Part model, mm, in its own coordinate system. A direction names the side the tool comes from. Coordinates: 2 decimals unless noted, no trailing zeros. Loops run counter-clockwise (first coordinate to the right, second up) from the corner with the lowest first, then second, coordinate; pieces in that order, holes last. Notation, with made-up numbers: M 58,59 L 105,59 A25 cw 105,93 Z; hole C 37.25,22.25 d2. An arc over 180 degrees is marked long. Use a Markdown table: item, result. Add a question column.
1) Pin check, flat tips, straight feed: pin 1 Ø9.5 at (x, y) = (-57, -0.5) entering from +Z; pin 2 Ø6 at (x, y) = (-46.5, 99) entering from +Z; pin 3 Ø10 at (x, y) = (-109.5, 230) entering from -Z. Stop position of each tip, or through.
2) Band-saw the part on D-D (y = 132.5). List the corners of the cut face in (x, z).
3) Band-saw the part on B-B (x = -59.69). List the corners of the cut face in (y, z) (3 decimals), plus the area to 3 significant figures.
4) Tool access for faces 5 (the flat face through (342.9, 253, 42)), 6 (the cylindrical face through (50.605, -2.861, 18.21)), 7 (the flat face through (-293, 203.2, 54)), 8 (the cylindrical face through (-248.94, 254.71, 89.28)): list every direction of +Z, -Z, +X, -X, +Y, -Y with a clear straight run to the whole face (end or side of a thin tool).
5) Wall check: probe 1 along X at (y, z) = (184, -64); probe 2 along Y at (x, z) = (0, 12.5); probe 3 along X at (y, z) = (284.5, 32.5). Give the ranges that are in metal, low to high. Write a range as from..to.
6) Band-saw the part on A-A (z = -78.5). List the corners of the cut face in (x, y), plus the area to 3 significant figures.
7) Band-saw the part on C-C (y = 59.69). List the corners of the cut face in (x, z) (3 decimals), plus the area to 3 significant figures.
8) Pull direction X, two halves, no side cores. Call faces 1 (the cylindrical face through (-248.94, -62.79, 89.28)), 2 (the flat face through (-342.9, 253, 42)), 3 (the flat face through (-293, -12.7, 54)), 4 (the flat face through (-6, 98, 0)): released by +X, released by -X, zero draft, split by the parting line, or undercut.
from build123d import *

# Parameters (mm, degrees)
F0_W     = 914.4
F0_H     = 419.1
F1_DEPTH = 12.7
F2_R     = 36.83
F3_DEPTH = 12.7
F4_R     = 9.525
F5_DEPTH = 11.176
F6_W     = 101.6
F6_H     = 101.6
F7_DEPTH = 83.82
F8_W     = 12.7
F8_H     = 419.1
F9_DEPTH = 254
F10_R    = 25.4


with BuildPart() as f1:
    # F0 (on Top) → F1 (new body)
    with BuildSketch(Plane.XY):
        with Locations((0, 95.25)):
            Rectangle(F0_W, F0_H)
    extrude(amount=F1_DEPTH)

    # F2 (on face) → F3 (cut)
    with BuildSketch(Plane.XY.offset(12.7)):
        Circle(F2_R)
    extrude(amount=-F3_DEPTH, mode=Mode.SUBTRACT)

    # F4 (on face) → F5 (join)
    with BuildSketch(Plane.XY.offset(12.7)):
        with BuildLine():
            ThreePointArc((9.525, 59.69), (-6.7351920908, 66.4251920908), (0, 50.165))
            ThreePointArc((0, 50.165), (6.7351920908, 52.9548079092), (9.525, 59.69))
        make_face()
        with BuildLine():
            Line((36.83, 0), (48.26, 0))
            ThreePointArc((48.26, 0), (34.1249732601, 34.1249732601), (0, 48.26))
            Line((0, 48.26), (0, 36.83))
            ThreePointArc((0, 36.83), (26.0427427511, 26.0427427511), (36.83, 0))
        make_face()
        with BuildLine():
            Line((0, 36.83), (0, 48.26))
            ThreePointArc((0, 48.26), (-34.1249732601, 34.1249732601), (-48.26, 0))
            Line((-48.26, 0), (-36.83, 0))
            ThreePointArc((-36.83, 0), (-26.0427427511, 26.0427427511), (0, 36.83))
        make_face()
        with BuildLine():
            ThreePointArc((-48.26, 0), (-34.1249732601, -34.1249732601), (0, -48.26))
            Line((0, -48.26), (0, -36.83))
            ThreePointArc((0, -36.83), (-26.0427427511, -26.0427427511), (-36.83, 0))
            Line((-36.83, 0), (-48.26, 0))
        make_face()
        with BuildLine():
            ThreePointArc((0, -48.26), (34.1249732601, -34.1249732601), (48.26, 0))
            Line((48.26, 0), (36.83, 0))
            ThreePointArc((36.83, 0), (26.0427427511, -26.0427427511), (0, -36.83))
            Line((0, -36.83), (0, -48.26))
        make_face()
        with Locations((-59.69, 0)):
            Circle(F4_R)
        with BuildLine():
            ThreePointArc((9.525, -59.69), (6.7351920908, -52.9548079092), (0, -50.165))
            ThreePointArc((0, -50.165), (-6.7351920908, -66.4251920908), (9.525, -59.69))
        make_face()
        with BuildLine():
            ThreePointArc((69.215, 0), (59.69, 9.525), (50.165, 0))
            ThreePointArc((50.165, 0), (59.69, -9.525), (69.215, 0))
        make_face()
    extrude(amount=F5_DEPTH)

    # F6 (on face) → F7 (join)
    with BuildSketch(Plane.XY.offset(12.7)):
        with Locations((-292.1, 254)):
            Rectangle(F6_W, F6_H)
        with Locations((-292.1, -63.5)):
            Rectangle(F6_W, F6_H)
        with Locations((292.1, -63.5)):
            Rectangle(F6_W, F6_H)
        with Locations((292.1, 254)):
            Rectangle(F6_W, F6_H)
    extrude(amount=F7_DEPTH)

    # F8 (on face) → F9 (join)
    with BuildSketch(Plane(origin=(0, 0, 0), x_dir=(1, 0, 0), z_dir=(0, 0, -1))):
        with Locations((-450.85, -95.25)):
            Rectangle(F8_W, F8_H)
        with Locations((450.85, -95.25)):
            Rectangle(F8_W, F8_H)
    extrude(amount=F9_DEPTH)

    # F10
    f10_edges = [f1.edges().sort_by_distance(p)[0] for p in [
        (-342.9, -63.5, 96.52),
        (-342.9, 254, 96.52),
        (-241.3, 254, 96.52),
        (-241.3, -63.5, 96.52),
        (241.3, -63.5, 96.52),
        (241.3, 254, 96.52),
        (342.9, 254, 96.52),
        (342.9, -63.5, 96.52),
    ]]
    fillet(f10_edges, radius=F10_R)


solid = f1.part
Entries:
| question | item | result |
|---|---|---|
| 1 | pin 1 | z = 23.88 |
| 1 | pin 2 | z = 12.7 |
| 1 | pin 3 | z = 0 |
| 2 | outline | M -457.2,-254 L -444.5,-254 L -444.5,0 L 444.5,0 L 444.5,-254 L 457.2,-254 L 457.2,12.7 L -457.2,12.7 Z |
| 3 | outline | M -114.3,0 L 304.8,0 L 304.8,12.7 L 9.525,12.7 L 9.525,23.876 L -9.525,23.876 L -9.525,12.7 L -114.3,12.7 Z |
| 3 | area | 5,540 mm2 |
| 4 | face 5 | +Z, +X, +Y, -Y |
| 4 | face 6 | +Z |
| 4 | face 7 | +Z, +X, -X |
| 4 | face 8 | +Z, +Y, -Y |
| 5 | probe 1 | -457.2..-444.5, 444.5..457.2 |
| 5 | probe 2 | -114.3..-36.83, 36.83..304.8 |
| 5 | probe 3 | -342.9..-241.3, 241.3..342.9 |
| 6 | outline | M -457.2,-114.3 L -444.5,-114.3 L -444.5,304.8 L -457.2,304.8 Z; M 444.5,-114.3 L 457.2,-114.3 L 457.2,304.8 L 444.5,304.8 Z |
| 6 | area | 10,600 mm2 |
| 7 | outline | M -457.2,-254 L -444.5,-254 L -444.5,0 L 444.5,0 L 444.5,-254 L 457.2,-254 L 457.2,12.7 L 9.525,12.7 L 9.525,23.876 L -9.525,23.876 L -9.525,12.7 L -457.2,12.7 Z |
| 7 | area | 18,300 mm2 |
| 8 | face 1 | undercut |
| 8 | face 2 | released by -X |
| 8 | face 3 | zero draft |
| 8 | face 4 | undercut |
